```python
from build123d import *

# Parameters (mm, degrees)
F1_ANGLE = 180


with BuildPart() as f1:
    # F0 (on Front) → F1 (revolve)
    with BuildSketch(Plane.XZ):
        with BuildLine():
            ThreePointArc((-34.095638, 0), (-20.558778, 17.018454), (0, 24.104428))
            Line((0, 24.104428), (-0.046644, 25.103341))
            ThreePointArc((-0.046644, 25.103341), (-21.735137, 17.403096), (-35.555795, -1))
            Line((-35.555795, -1), (-11.48195, -1))
            Line((-11.48195, -1), (-11.48195, -16.015298))
            Line((-11.48195, -16.015298), (-10.48195, -16.015298))
            Line((-10.48195, -16.015298), (-10.48195, 0))
            Line((-10.48195, 0), (-34.095638, 0))
        make_face()
    revolve(axis=Axis((0, 0, 5.296746), (0, 0, -1)), revolution_arc=F1_ANGLE)


solid = f1.part
```
Work out the finished part from the listing and answer in its coordinate system (mm). A direction names the side the tool comes from. Coordinates: 2 decimals unless noted, no trailing zeros. Loops run counter-clockwise (first coordinate to the right, second up) from the corner with the lowest first, then second, coordinate; pieces in that order, holes last.
1) Section A-A (z = -5) is taken. Give the vertices of the cut face in (x, y).
Results:
outline: (-11.48, 0) - (-10.48, 0) arc R10.48 cw to (10.48, 0) - (11.48, 0) arc R11.48 ccw to start
2) For faces 1 (the cylindrical face through (-0.23, 10.48, -7.9)), 2 (the flat face through (0, 17, 0)), 3 (the flat face through (0, 18, -1)), determine the directions among +Z, -Z, +X, -X, +Y, -Y from which every point of the face is accessible in a straight line to the end or side of a thin tool.
Results:
face 1: -Z, -Y
face 2: -Y
face 3: -Z, +Y
3) Consider probe 1 along Z at (x, y) = (24, 2.5); probe 2 along Z at (x, y) = (23, 9.5); probe 3 along X at (y, z) = (26, 3). Determine where each line is inside the solid, lowest interval first.
Results:
probe 1: z = -1 to 0, 14.16 to 15.5
probe 2: z = -1 to 0, 13.47 to 14.83
probe 3: x = -21.65 to -19.86, 19.86 to 21.65
4) Flat-ended cylindrical pins translate along their axes: pin 1 (4 mm diameter, centred on y = 9, z = 2.5, fed in from +X); pin 2 (5 mm diameter, centred on x = 7, z = 6.5, fed in from +Y); pin 3 (12 mm diameter, centred on x = 13, y = 23.5, fed in from +Z). Find the tip coordinate at first contact, or state that the pin passes through.
Results:
pin 1: stops at x = 33.93
pin 2: stops at y = 32.67
pin 3: stops at z = 18.03
